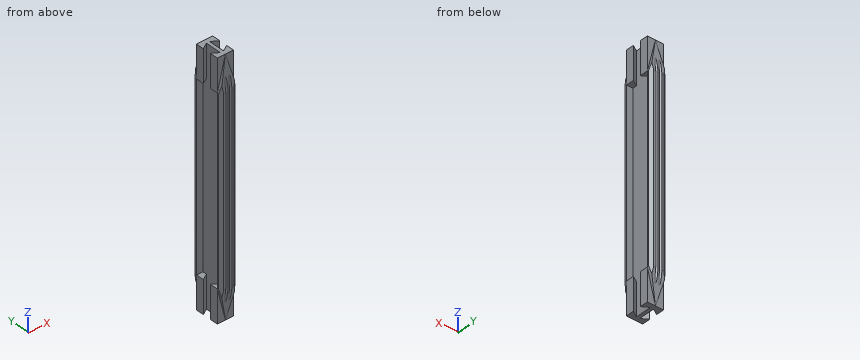
from build123d import *

# Parameters (mm, degrees)
SKETCH1_W               = 152
SKETCH1_H               = 15
BOSS_EXTRUDE1_DEPTH     = 1
SKETCH2_W               = 20
SKETCH2_H               = 15
BOSS_EXTRUDE2_DEPTH     = 4
CUT_EXTRUDE1_DEPTH      = 133.3074072
MIRROR2_COPY_1_SKETCH_W = 20
MIRROR2_COPY_1_SKETCH_H = 15
MIRROR2_COPY_1_DEPTH    = 4
MIRROR2_COPY_2_DEPTH    = 133.3074072
BOSS_EXTRUDE5_DEPTH     = 2.5
CUT_EXTRUDE2_DEPTH      = 78.30459236
SKETCH9_R               = 0.75
CUT_EXTRUDE3_DEPTH      = 153.410629551
CUT_EXTRUDE4_DEPTH      = 153.410629551


with BuildPart() as part:
    # Sketch1 → Boss-Extrude1 (new, symmetric)
    with BuildSketch(Plane(origin=(0, 0, 0), x_dir=(0, 0, -1), z_dir=(1, 0, 0))):
        Rectangle(SKETCH1_W, SKETCH1_H)
    extrude(amount=BOSS_EXTRUDE1_DEPTH, both=True)

    # Sketch2 → Boss-Extrude2 (add)
    with BuildSketch(Plane(origin=(1, 0, 0), x_dir=(0, 0, -1), z_dir=(1, 0, 0))):
        with Locations((66, 0)):
            Rectangle(SKETCH2_W, SKETCH2_H)
    boss_extrude2 = extrude(amount=BOSS_EXTRUDE2_DEPTH)

    # Sketch3 → Cut-Extrude1 (cut, through all)
    with BuildSketch(Plane.XY.offset(-56)):
        Polygon((5, 2.5), (1, 5), (1, -5), (5, -2.5), align=None)
    cut_extrude1 = extrude(amount=-CUT_EXTRUDE1_DEPTH, mode=Mode.SUBTRACT)

    # Mirror1: Boss-Extrude2, Cut-Extrude1 across plane
    add(boss_extrude2.mirror(Plane(origin=(0, 0, 0), x_dir=(0, 0, 1), z_dir=(1, 0, 0))))
    add(cut_extrude1.mirror(Plane(origin=(0, 0, 0), x_dir=(0, 0, 1), z_dir=(1, 0, 0))), mode=Mode.SUBTRACT)

    # Mirror2: Boss-Extrude2, Cut-Extrude1 across plane
    add(boss_extrude2.mirror(Plane.XY))
    add(cut_extrude1.mirror(Plane.XY), mode=Mode.SUBTRACT)

    # Mirror2 copy 1 sketch → Mirror2 copy 1 (add)
    with BuildSketch(Plane.ZY.offset(1)):
        with Locations((66, 0)):
            Rectangle(MIRROR2_COPY_1_SKETCH_W, MIRROR2_COPY_1_SKETCH_H)
    extrude(amount=MIRROR2_COPY_1_DEPTH)

    # Mirror2 copy 2 sketch → Mirror2 copy 2 (cut, through all)
    with BuildSketch(Plane(origin=(0, 0, 56), x_dir=(-1, 0, 0), z_dir=(0, 0, -1))):
        Polygon((5, 2.5), (1, 5), (1, -5), (5, -2.5), align=None)
    extrude(amount=-MIRROR2_COPY_2_DEPTH, mode=Mode.SUBTRACT)

    # Sketch7 → Boss-Extrude5 (add)
    with BuildSketch(Plane(origin=(0, 7.5, 0), x_dir=(1, 0, 0), z_dir=(0, 1, 0))):
        Polygon((0, -76), (-5, -56), (-5, 56), (0, 76), (5, 56), (5, -56), align=None)
    boss_extrude5 = extrude(amount=BOSS_EXTRUDE5_DEPTH)

    # Sketch8 → Cut-Extrude2 (cut, through all)
    with BuildSketch(Plane.ZY.offset(5)):
        Polygon((-56, 10), (-76, 7.5), (-76, 10), align=None)
        Polygon((76, 10), (56, 10), (76, 7.5), align=None)
    cut_extrude2 = extrude(amount=-CUT_EXTRUDE2_DEPTH, mode=Mode.SUBTRACT)

    # Sketch9 → Cut-Extrude3 (cut, through all)
    with BuildSketch(Plane.XY.offset(76)):
        with Locations((1.2, 9.7)):
            Circle(SKETCH9_R)
        with Locations((-1.2, 9.7)):
            Circle(SKETCH9_R)
    cut_extrude3 = extrude(amount=-CUT_EXTRUDE3_DEPTH, mode=Mode.SUBTRACT)

    # Mirror4: Boss-Extrude5, Cut-Extrude2, Cut-Extrude3 across plane
    add(boss_extrude5.mirror(Plane.ZX))
    add(cut_extrude2.mirror(Plane.ZX), mode=Mode.SUBTRACT)
    add(cut_extrude3.mirror(Plane.ZX), mode=Mode.SUBTRACT)

    # Sketch10 → Cut-Extrude4 (cut, through all)
    with BuildSketch(Plane(origin=(0, 0, -76), x_dir=(-1, 0, 0), z_dir=(0, 0, -1))):
        Polygon((-5, 8.5), (-3.2, 10), (-5, 10), align=None)
        Polygon((5, 10), (5, 8.5), (3.2, 10), align=None)
        Polygon((-5, -10), (-5, -8.5), (-3.2, -10), align=None)
        Polygon((5, -8.5), (3.2, -10), (5, -10), align=None)
    extrude(amount=-CUT_EXTRUDE4_DEPTH, mode=Mode.SUBTRACT)


solid = part.part
Check sheet for the modelled part. Datum: model origin and axes. Units: mm. Coordinates: 2 decimals unless noted, no trailing zeros. Loops run counter-clockwise (first coordinate to the right, second up) from the corner with the lowest first, then second, coordinate; pieces in that order, holes last. Notation, with made-up numbers: (86, 28.5) -> (117, 28.5) arc R34 cw to (117, 63.5) -> close; hole circle Ø8 at (11.5, -28). An arc over 180 degrees is marked (long way). Write item = value, one per line. Start each with the question number.
1. Section check A-A on z = 33.5. Record the cut outline in (x, y), then the cut area to 3 significant figures.
2. Material ranges on line 1 (Y direction, x = -2.75, z = 45); line 2 (X direction, y = 9.7, z = 3); line 3 (Y direction, x = 1.2, z = 8), recorded low to high.
3. Section check B-B on y = -3.75. Record the cut outline in (x, z), then the cut area to 3 significant figures.
4. Depth check by flat-ended pin: P1, Ø0.9, axis at x = 1.2, y = -9.7, coming from the +Z side; P2, Ø3, axis at y = -5.5, z = 36, coming from the -X side; P3, Ø2.5, axis at x = -1.5, z = 68, coming from the +Y side; P4, Ø4, axis at x = 2.5, z = -65.5, coming from the -Y side. Enter the tip coordinate at first touch or a pass-through.
Responses:
q1.outline = (-5, -8.5) -> (-3.2, -10) -> (-1.89, -10) arc R0.75 cw (long way) to (-0.51, -10) -> (0.51, -10) arc R0.75 cw (long way) to (1.89, -10) -> (3.2, -10) -> (5, -8.5) -> (5, -7.5) -> (1, -7.5) -> (1, 7.5) -> (5, 7.5) -> (5, 8.5) -> (3.2, 10) -> (1.89, 10) arc R0.75 cw (long way) to (0.51, 10) -> (-0.51, 10) arc R0.75 cw (long way) to (-1.89, 10) -> (-3.2, 10) -> (-5, 8.5) -> (-5, 7.5) -> (-1, 7.5) -> (-1, -7.5) -> (-5, -7.5) -> close
q1.area = 69.3 mm2
q2.line_1 = -10 to -7.5, 7.5 to 10
q2.line_2 = -3.56 to -1.95, -0.45 to 0.45, 1.95 to 3.56
q2.line_3 = -8.95 to -7.5, 7.5 to 8.95
q3.outline = (-5, -76) -> (-3, -76) -> (-3, -56) -> (-5, -56) -> close; (-5, 56) -> (-3, 56) -> (-3, 76) -> (-5, 76) -> close; (-1, -76) -> (1, -76) -> (1, 76) -> (-1, 76) -> close; (3, -76) -> (5, -76) -> (5, -56) -> (3, -56) -> close; (3, 56) -> (5, 56) -> (5, 76) -> (3, 76) -> close
q3.area = 464 mm2
q4.P1 = through
q4.P2 = -1
q4.P3 = 8.66
q4.P4 = -9.06
